Input: part model. Units: mm. Frame: model coordinates. Round coordinates to 2 decimals unless told otherwise and drop trailing zeros. Order: outer loops, then holes, each group sorted by start corner. A loop starts at its lowest first (then second) coordinate and runs counter-clockwise, first axis right, second up. Notation, with made-up numbers: M 65,80.5 L 101,80.5 A24 ccw 101,102.5 Z; hole C 44.25,-23 d4. An arc over 180 degrees is marked long. One line per question, with ' | ' between items.
```python
from build123d import *

# Parameters (mm, degrees)
ESQUISSE1_R             = 52.5
BOSS_EXTRU_1_DEPTH      = 50
ESQUISSE2_R             = 51
ENL_V_MAT_EXTRU_1_DEPTH = 90.51256895
ENL_V_MAT_EXTRU_2_DEPTH = 90.51256895


with BuildPart() as part:
    # Esquisse1 → Boss.-Extru.1 (new body)
    with BuildSketch(Plane.XY):
        Circle(ESQUISSE1_R)
    extrude(amount=BOSS_EXTRU_1_DEPTH)

    # Esquisse2 → Enlèv. mat.-Extru.1 (cut, through all)
    with BuildSketch(Plane.XY.offset(50)):
        Circle(ESQUISSE2_R)
    extrude(amount=-ENL_V_MAT_EXTRU_1_DEPTH, mode=Mode.SUBTRACT)

    # Esquisse3 → Enlèv. mat.-Extru.2 (cut, through all)
    with BuildSketch(Plane.XY.offset(50)):
        Polygon((-297.287137637, 0), (-52.5, 0), (52.5, 0), (297.287137637, 0), (297.287137637, 489.574275275), (-297.287137637, 489.574275275), align=None)
    extrude(amount=-ENL_V_MAT_EXTRU_2_DEPTH, mode=Mode.SUBTRACT)


solid = part.part
```
Item 1: First-contact query: pin 1 (12 mm diameter, centred on x = -38.5, z = 32.5, fed in from +Y); pin 2 (1 mm diameter, centred on x = -9.5, z = 6.5, fed in from -Y); pin 3 (10 mm diameter, centred on y = -9.5, z = 37, fed in from -X). Flat tips, straight axial feed; report the tip coordinate or a pass-through.
Report:
pin 1: y = -24.91 | pin 2: y = -51.72 | pin 3: x = -52.31
Item 2: Section query B-B, the plane y = -13.5. Return loops of the section in (x, z), plus the area to 3 significant figures.
Report:
outline: M -50.73,0 L -49.18,0 L -49.18,50 L -50.73,50 Z; M 49.18,0 L 50.73,0 L 50.73,50 L 49.18,50 Z | area: 155 mm²
Item 3: Mould query, pull axis X, two halves, no side actions, for faces 1 (the cylindrical face through (-1.121, -50.988, 25.35)), 2 (the cylindrical face through (-1.154, -52.487, 24.65)), 3 (the flat face through (-4, -51, 0)). Classes: +X half, -X half, draft (parallel to the pull), parting line (faces both ways), or undercut.
Report:
face 1: undercut | face 2: parting line | face 3: draft
Item 4: Section query A-A, the plane y = -49. Return loops of the section in (x, z), plus the area to 3 significant figures.
Report:
outline: M -18.85,0 L -14.14,0 L -14.14,50 L -18.85,50 Z; M 14.14,0 L 18.85,0 L 18.85,50 L 14.14,50 Z | area: 471 mm²
Item 5: Line query: line 1 along X through (y, z) = (-21, 36.5); line 2 along X through (y, z) = (-27.5, 47.5); line 3 along Y through (x, z) = (18, 36.5). Output: solid intervals per line, ascending. Write a range as from..to.
Report:
line 1: -48.12..-46.48, 46.48..48.12 | line 2: -44.72..-42.95, 42.95..44.72 | line 3: -49.32..-47.72
Item 6: Section query C-C, the plane z = 36.5. Return loops of the section in (x, y).
Report:
outline: M -52.5,0 A52.5 ccw 52.5,0 L 51,0 A51 cw -51,0 Z
Item 7: Section query D-D, the plane x = -19. Return loops of the section in (y, z), plus the area to 3 significant figures.
Report:
outline: M -48.94,0 L -47.33,0 L -47.33,50 L -48.94,50 Z | area: 80.6 mm²
